```python
from build123d import *

# Parameters (mm, degrees)
F3_COUNT = 4
F4_R     = 10.234547
F5_DEPTH = 25
F6_R     = 10.834547
F6_R_2   = 10.234547
F7_DEPTH = 3


with BuildPart() as f2:
    # F1 (on Front) → F2 section 0
    with BuildSketch(Plane.XZ, mode=Mode.PRIVATE) as f2_s0:
        Polygon((0, 4), (-15, 0), (15, 0), align=None)
    loft([f2_s0.sketch, Vertex(0, -40, 0)])

    # F3: F2 ×4 about axis
    f3_axis = Axis((0, 0, 1.111546), (0, 0, 1))


with BuildPart() as f2_1:
    add(f2.part)
    for i in range(1, F3_COUNT):
        add(f2.part.rotate(f3_axis, i * 360 / F3_COUNT))

    # F4 (on Top) → F5 (cut)
    with BuildSketch(Plane.XY):
        Circle(F4_R)
    extrude(amount=F5_DEPTH, mode=Mode.SUBTRACT)

    # F6 (on Top) → F7 (join)
    with BuildSketch(Plane.XY):
        Circle(F6_R)
        Circle(F6_R_2, mode=Mode.SUBTRACT)
    extrude(amount=F7_DEPTH)

    # F8: F2 across plane


with BuildPart() as f2_2:
    add(f2_1.part)
    add(f2_1.part.mirror(Plane.XY))


solid = f2_2.part
```
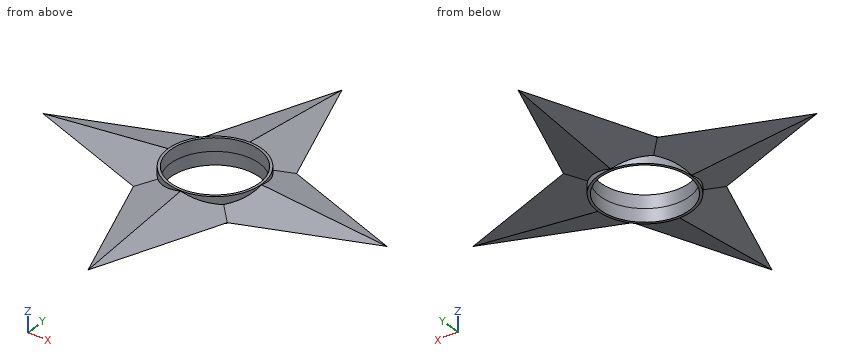
CAD build for the part. Positions are in the model's coordinates, mm. Give positions to 0.01 mm unless a question says otherwise; leave off trailing zeros. Order: outer loops, then holes, each group sorted by start corner. A loop starts at its lowest first (then second) coordinate and runs counter-clockwise, first axis right, second up.
(1) Flat gauge pin, fed straight in: pin 1 (4 mm diameter, centred on x = 19, y = 6, fed in from -Z). Where does the tip first touch, or does it go through?
(2) Saw through at D-D, the plane y = 14. Give the cut face in (x, z), then the cut area to 3 significant figures.
(3) Saw through at C-C, the plane y = 5. Give the cut face in (x, z).
(4) Saw through at B-B, the plane x = 18. Give the cut face in (y, z), then the cut area to 3 significant figures.
(5) Drill centre lines: L1, parallel to Z at x = -4, y = -18; L2, parallel to Z at x = 6.5, y = 9. Where is each one in solid material? Low to high.
(6) Saw through at A-A, the plane y = -6. Give the cut face in (x, z).
Results found:
1. pin 1: stops at z = -1.07
2. outline: (-9.75, 0) - (0, -2.6) - (9.75, 0) - (0, 2.6) - close
2. area: 50.7 mm2
3. outline: (-26.67, 0) - (-9.61, -1.71) - (-9.61, -3) - (-8.93, -3) - (-8.93, 3) - (-9.61, 3) - (-9.61, 1.71) - close; (8.93, -3) - (9.61, -3) - (9.61, -1.71) - (26.67, 0) - (9.61, 1.71) - (9.61, 3) - (8.93, 3) - close
4. outline: (-8.25, 0) - (0, -2.2) - (8.25, 0) - (0, 2.2) - close
4. area: 36.3 mm2
5. L1: z = -1.13 to 1.13
5. L2: z = -1.37 to 1.37
6. outline: (-24, 0) - (-9.02, -1.5) - (-9.02, -3) - (-8.29, -3) - (-8.29, 3) - (-9.02, 3) - (-9.02, 1.5) - close; (8.29, -3) - (9.02, -3) - (9.02, -1.5) - (24, 0) - (9.02, 1.5) - (9.02, 3) - (8.29, 3) - close
